```python
from build123d import *

# Parameters (mm, degrees)
SKETCH3_R               = 42
SKETCH3_R_2             = 40
BOSS_EXTRUDE1_DEPTH     = 905
CUT_EXTRUDE1_REACH      = 464.143
CUT_EXTRUDE1_END_RADIUS = 40
SKETCH4_R               = 3
CIRPATTERN1_COUNT       = 6


with BuildPart() as part:
    # Sketch3 → Boss-Extrude1 (new body)
    with BuildSketch(Plane.XY.offset(452.5)):
        Circle(SKETCH3_R)
        Circle(SKETCH3_R_2, mode=Mode.SUBTRACT)
    extrude(amount=-BOSS_EXTRUDE1_DEPTH)

    # Cut-Extrude1: up to this cylinder (the profile starts outside it)
    cut_extrude1_end = Plane(origin=(0, 0, 437.5), z_dir=(0, 0, 1)) * Cylinder(CUT_EXTRUDE1_END_RADIUS, 1009.286, mode=Mode.PRIVATE)
    # Sketch4 → Cut-Extrude1 (cut, up to the surface)
    with BuildSketch(Plane(origin=(42, 0, 0), x_dir=(0, 0, -1), z_dir=(1, 0, 0)), mode=Mode.PRIVATE) as cut_extrude1_sk1:
        with Locations((-437.5, 0)):
            Circle(SKETCH4_R)
    cut_extrude1_tool1 = extrude(cut_extrude1_sk1.sketch, amount=-CUT_EXTRUDE1_REACH, mode=Mode.PRIVATE) - cut_extrude1_end
    cut_extrude1 = cut_extrude1_tool1.solids().sort_by_distance((42, 0, 437.5))[0]
    add(cut_extrude1, mode=Mode.SUBTRACT)

    # CirPattern1: Cut-Extrude1 ×6 about axis
    cirpattern1_axis = Axis((0, 0, 452.5), (0, 0, 1))
    for i in range(1, CIRPATTERN1_COUNT):
        add(cut_extrude1.rotate(cirpattern1_axis, i * 360 / CIRPATTERN1_COUNT), mode=Mode.SUBTRACT)


solid = part.part
```
Geometry check sheet. Reference: the model listing, model coordinates, mm. Coordinates: 2 decimals unless noted, no trailing zeros. Write each loop counter-clockwise with the first axis right and the second up, starting at its lowest first coordinate (ties: lowest second). Pieces come first, ordered by that corner, then holes. Notation, with made-up numbers: (77.25, 60.5) -> (93.25, 60.5) arc R19 ccw to (93.25, 65.5) -> close; hole circle Ø7 at (54.5, 62). An arc over 180 degrees is marked (long way). Use CSV: the item, a comma, the result in double quotes. Start each with the question number.
Item 1: Thickness scan on line 1 (X direction, y = -13, z = 202); line 2 (Y direction, x = -1.5, z = 288); line 3 (Y direction, x = 2.5, z = 233). Record the ranges inside material, lowest first.
Item 2: Mould release check, pull along X, two halves, no side actions. Record for faces 1 (the cylindrical face through (-8.67, -39.05, 6.33)), 2 (the flat face through (37.1, -15.4, 452.5)), 3 (the cylindrical face through (40.06, 12.62, 6.33)): released by +X, released by -X, zero draft, split by the parting line, or undercut.
Item 3: Cross-section at A-A, the plane x = 0. Record the cut outline in (y, z).
Item 4: Depth check by flat-ended pin: pin 1 Ø3.5 at (y, z) = (0, 437.5) entering from +X; pin 2 Ø6 at (x, z) = (-29.5, -202) entering from +Y; pin 3 Ø1 at (y, z) = (-3, 132) entering from +X; pin 4 Ø10 at (y, z) = (8, 258.5) entering from -X. Enter the tip coordinate at first touch or a pass-through.
Item 5: Cross-section at B-B, the plane z = -87. Record the cut outline in (x, y).
Answers:
1,line 1,"-39.94 to -37.83, 37.83 to 39.94"
1,line 2,"-41.97 to -39.97, 39.97 to 41.97"
1,line 3,"-41.93 to -39.92, 39.92 to 41.93"
2,face 1,"undercut"
2,face 2,"zero draft"
2,face 3,"split by the parting line"
3,outline,"(-42, -452.5) -> (-40, -452.5) -> (-40, 452.5) -> (-42, 452.5) -> close; (40, -452.5) -> (42, -452.5) -> (42, 452.5) -> (40, 452.5) -> close"
4,pin 1,"through"
4,pin 2,"y = 32.58"
4,pin 3,"x = 41.93"
4,pin 4,"x = -41.89"
5,outline,"circle Ø84 at (0, 0); hole circle Ø80 at (0, 0)"
